Read the model definition and answer for the solid it produces. Units are mm, in the model's axes. Face numbers are marked on the shaded views. A direction names the side the tool comes from. Give positions to 0.01 mm unless a question says otherwise; leave off trailing zeros. Write each loop counter-clockwise with the first axis right and the second up, starting at its lowest first coordinate (ties: lowest second). Pieces come first, ordered by that corner, then holes. Notation, with made-up numbers: (-6.75, 36) -> (29.25, 36) arc R13 ccw to (29.25, 60) -> close; hole circle Ø10 at (88, 63). An arc over 180 degrees is marked (long way). Answer as CSV lines item,"result". Start each with the question number.
1. A tool of negligible diameter and unlimited length cuts with its end or side. For the marked faces 1, 2 and 3, from which of +Z, -Z, +X, -X, +Y, -Y can it reach the whole face along a straight path? Write none if from no direction.
2. The part is cut by section D-D, the plane x = -12.5. Determine the outline of the cut face in (y, z) (3 decimals), and give its area (3 significant figures).
3. Given pin 1 (4 mm diameter, centred on x = 22, y = 12.7, fed in from +Z); pin 2 (1 mm diameter, centred on x = 2.5, z = 6, fed in from -Y); pin 3 (1.5 mm diameter, centred on y = 20.5, z = 1.5, fed in from +X); pin 4 (1.5 mm diameter, centred on x = -5.5, z = 3, fed in from -Y), each flat-ended and moving along its own axis, determine where each tip first touches the part or whether it passes through.
4. The part is cut by section A-A, the plane y = 0. Determine the outline of the cut face in (x, z) (1 decimal), and give its area (3 significant figures).
5. The part is cut by section B-B, the plane z = 6. Determine the outline of the cut face in (x, y).
6. Find the intervals of material crossed by line 1 (X direction, y = 20.5, z = 1); line 2 (Z direction, x = -4.5, y = -27) (3 decimals); line 3 (Y direction, x = 0.5, z = 2.25), in increasing order.
7. The part is cut by section C-C, the plane y = -22. Determine the outline of the cut face in (x, z) (3 decimals), and give its area (3 significant figures).
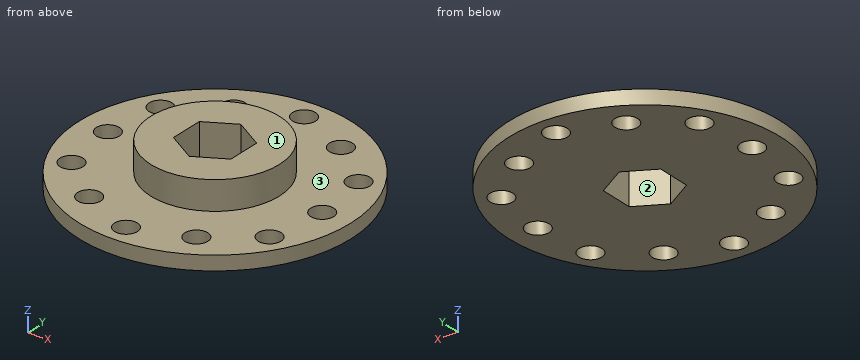
from build123d import *

# Parameters (mm, degrees)
SKETCH1_W           = 30.1625
SKETCH1_H           = 3.175
SKETCH2_R           = 14.2748
BOSS_EXTRUDE1_DEPTH = 6.35
CUT_EXTRUDE1_DEPTH  = 10.525
HOLE1_D             = 5.1054
HOLE1_DEPTH         = 9.525


with BuildPart() as part:
    # Sketch1 → Revolve1 (revolve)
    with BuildSketch(Plane(origin=(0, 0, 0), x_dir=(1, 0, 0), z_dir=(0, 1, 0))):
        with Locations((15.08125, -1.5875)):
            Rectangle(SKETCH1_W, SKETCH1_H)
    revolve(axis=Axis((0, 0, 0), (0, 0, 1)))

    # Sketch2 → Boss-Extrude1 (add)
    with BuildSketch(Plane.XY.offset(3.175)):
        Circle(SKETCH2_R)
    extrude(amount=BOSS_EXTRUDE1_DEPTH)

    # Sketch3 → Cut-Extrude1 (cut, through all)
    with BuildSketch(Plane.XY.offset(9.525)):
        Polygon((0, -7.361677812), (6.3754, -3.680838906), (6.3754, 3.680838906), (0, 7.361677812), (-6.3754, 3.680838906), (-6.3754, -3.680838906), align=None)
    extrude(amount=-CUT_EXTRUDE1_DEPTH, mode=Mode.SUBTRACT)

    # Hole1
    with Locations(Plane(origin=(0, 0, 0), x_dir=(-1, 0, 0), z_dir=(0, 0, -1))):
        with Locations((11.90625, 20.622229928), (0, 25.4), (23.8125, 0), (21.997045256, 12.7), (11.90625, -20.622229928), (21.997045256, -12.7), (-11.90625, -20.622229928), (0, -25.4), (-23.8125, 0), (-21.997045256, -12.7), (-11.90625, 20.622229928), (-21.997045256, 12.7)):
            Hole(HOLE1_D / 2, depth=HOLE1_DEPTH)


solid = part.part
Results found:
1,face 1,"+Z, +X, -X, +Y, -Y"
1,face 2,"+Z, -Z"
1,face 3,"+Z"
2,outline,"(-27.45, 0) -> (-23.105, 0) -> (-23.105, 3.175) -> (-27.45, 3.175) -> close; (-18.14, 0) -> (18.14, 0) -> (18.14, 3.175) -> (6.893, 3.175) -> (6.893, 9.525) -> (-6.893, 9.525) -> (-6.893, 3.175) -> (-18.14, 3.175) -> close; (23.105, 0) -> (27.45, 0) -> (27.45, 3.175) -> (23.105, 3.175) -> close"
2,area,"230 mm²"
3,pin 1,"passes through"
3,pin 2,"stops at y = -14.13"
3,pin 3,"stops at x = 22.8"
3,pin 4,"stops at y = -29.79"
4,outline,"(-30.2, 0) -> (-26.4, 0) -> (-26.4, 3.2) -> (-30.2, 3.2) -> close; (-21.3, 0) -> (-6.4, 0) -> (-6.4, 9.5) -> (-14.3, 9.5) -> (-14.3, 3.2) -> (-21.3, 3.2) -> close; (6.4, 0) -> (21.3, 0) -> (21.3, 3.2) -> (14.3, 3.2) -> (14.3, 9.5) -> (6.4, 9.5) -> close; (26.4, 0) -> (30.2, 0) -> (30.2, 3.2) -> (26.4, 3.2) -> close"
4,area,"219 mm²"
5,outline,"circle Ø28.55 at (0, 0); hole (-6.38, -3.68) -> (0, -7.36) -> (6.38, -3.68) -> (6.38, 3.68) -> (0, 7.36) -> (-6.38, 3.68) -> close"
6,line 1,"x = -22.13 to -14.46, -9.36 to 9.36, 14.46 to 22.13"
6,line 2,"z = 0 to 3.175"
6,line 3,"y = -30.16 to -27.9, -22.9 to -7.07, 7.07 to 22.9, 27.9 to 30.16"
7,outline,"(-20.634, 0) -> (-14.055, 0) -> (-14.055, 3.175) -> (-20.634, 3.175) -> close; (-9.757, 0) -> (9.757, 0) -> (9.757, 3.175) -> (-9.757, 3.175) -> close; (14.055, 0) -> (20.634, 0) -> (20.634, 3.175) -> (14.055, 3.175) -> close"
7,area,"104 mm²"
